```python
from build123d import *

# Parameters (mm, degrees)
F1_DEPTH = 38.1
F0_W     = 31.75
F0_H     = 12.7
F2_DEPTH = 25.4


with BuildPart() as f1:
    # F0 (on Top) → F1 (new body)
    with BuildSketch(Plane.XY):
        Polygon((63.5, 0), (0, 0), (0, -12.7), (31.75, -12.7), (63.5, -12.7), align=None)
    extrude(amount=F1_DEPTH)

    # F0 (on Top) → F2 (join)
    with BuildSketch(Plane.XY):
        Polygon((63.5, 0), (0, 0), (0, -12.7), (31.75, -12.7), (63.5, -12.7), align=None)
        with Locations((15.875, -19.05)):
            Rectangle(F0_W, F0_H)
    extrude(amount=F2_DEPTH)


solid = f1.part
```
Can you work these out from the model? Positions are in its coordinate system, mm. A direction names the side the tool comes from. Coordinates: 2 decimals unless noted, no trailing zeros. Order: outer loops, then holes, each group sorted by start corner. A loop starts at its lowest first (then second) coordinate and runs counter-clockwise, first axis right, second up.
1. For faces 1 (the face through (31.75, -19, 13)), 2 (the face through (16, -25.4, 13)), 3 (the face through (16, -19, 25.4)), which set-ups out of +Z, -Z, +X, -X, +Y, -Y let a thin tool reach every point of the face, with its end or its side?
2. If we section it at D-D (z = 33.5): Please give me the cut outline in (x, y).
3. I'm going to push flat-ended pins straight in: pin 1 (10 mm diameter, centred on y = -18, z = 13, fed in from +X); pin 2 (6.5 mm diameter, centred on x = 22, y = -20.5, fed in from +Z); pin 3 (1 mm diameter, centred on x = 50.5, z = 29, fed in from -Y). Where does each tip first touch, or does it pass through?
4. If we section it at C-C (y = -13.5): Please give me the cut outline in (x, z).
5. I need wall thicknesses on line 1 (Y direction, x = 12, z = 34); line 2 (X direction, y = -13, z = 4); line 3 (Z direction, x = 17, y = -18.5). Which ranges of each line are inside material? Lowest first, please.
6. If we section it at A-A (z = 18.5): Please give me the cut outline in (x, y), then the cut area to 3 significant figures.
7. If we section it at B-B (x = 6): Please give me the cut outline in (y, z), then the cut area to 3 significant figures.
Entries:
1. face 1: +Z, -Z, +X, -Y
1. face 2: +Z, -Z, +X, -X, -Y
1. face 3: +Z, +X, -X, -Y
2. outline: (0, -12.7) - (63.5, -12.7) - (63.5, 0) - (0, 0) - close
3. pin 1: stops at x = 31.75
3. pin 2: stops at z = 25.4
3. pin 3: stops at y = -12.7
4. outline: (0, 0) - (31.75, 0) - (31.75, 25.4) - (0, 25.4) - close
5. line 1: y = -12.7 to 0
5. line 2: x = 0 to 31.75
5. line 3: z = 0 to 25.4
6. outline: (0, -25.4) - (31.75, -25.4) - (31.75, -12.7) - (63.5, -12.7) - (63.5, 0) - (0, 0) - close
6. area: 1,210 mm2
7. outline: (-25.4, 0) - (0, 0) - (0, 38.1) - (-12.7, 38.1) - (-12.7, 25.4) - (-25.4, 25.4) - close
7. area: 806 mm2
